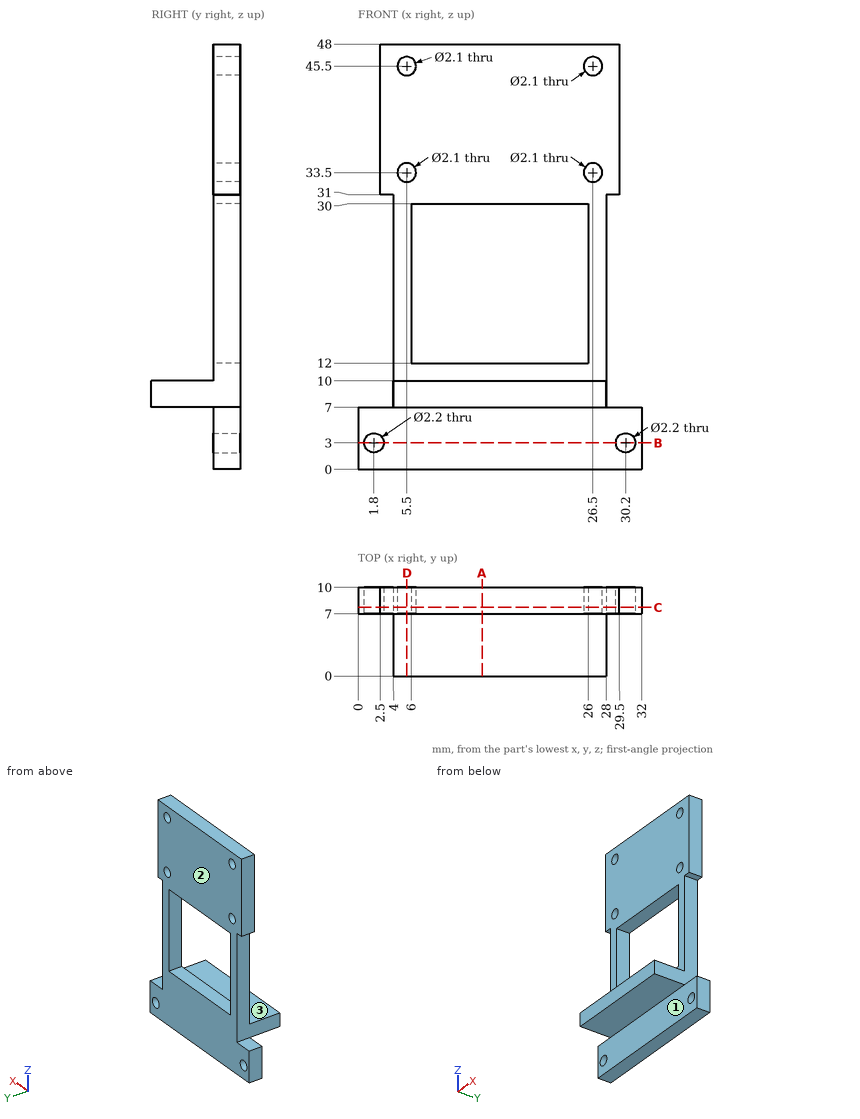
Part print with two shaded views. Sizes in mm from the minimum x, y, z corner. A direction names the side the tool comes from. Round coordinates to 2 decimals unless told otherwise and drop trailing zeros. Write each loop counter-clockwise with the first axis right and the second up, starting at its lowest first coordinate (ties: lowest second). Pieces come first, ordered by that corner, then holes. Notation, with made-up numbers: M 36.5,82.5 L 85.5,82.5 A5 cw 85.5,86.5 Z; hole C -4.5,68.5 d1. An arc over 180 degrees is marked long. Put each result on its own line as item: value. Start each with the question number.
1) Saw through at C-C, the plane y = 7.75. Write the cut outline in (x, z).
2) Pin check, flat tips, straight feed: pin 1 Ø1.7 at (x, z) = (26.5, 45.5) entering from -Y; pin 2 Ø5 at (y, z) = (8.5, 41.5) entering from +X; pin 3 Ø3.5 at (x, y) = (11.5, 2) entering from +Z; pin 4 Ø13.5 at (x, z) = (19, 24.5) entering from -Y. Stop position of each tip, or through.
3) Drill centre lines: probe 1 along Z at (x, y) = (26.5, 8); probe 2 along X at (y, z) = (8.3, 3); probe 3 along X at (y, z) = (8.3, 33.5). Where is each one in solid material? Low to high. Write a range as [from, to].
4) 3-axis set-ups, long thin cutter, end or side, ignore diameter. For the marked faces 1, 2 and 3: which of +Z, -Z, +X, -X, +Y, -Y reach the whole face in a straight line?
5) Saw through at A-A, the plane x = 14. Write the cut outline in (y, z).
6) Saw through at D-D, the plane x = 5.5. Write the cut outline in (y, z), and give its area (3 significant figures).
7) Saw through at B-B, the plane z = 3. Write the cut outline in (x, y).
Resolved:
1. outline: M 0,0 L 32,0 L 32,7 L 28,7 L 28,31 L 29.5,31 L 29.5,48 L 2.5,48 L 2.5,31 L 4,31 L 4,7 L 0,7 Z; hole C 1.8,3 d2.2; hole C 5.5,33.5 d2.1; hole C 5.5,45.5 d2.1; hole M 6,12 L 26,12 L 26,30 L 6,30 Z; hole C 26.5,33.5 d2.1; hole C 26.5,45.5 d2.1; hole C 30.2,3 d2.2
2. pin 1: through
2. pin 2: x = 29.5
2. pin 3: z = 10
2. pin 4: y = 7
3. probe 1: [0, 32.45], [34.55, 44.45], [46.55, 48]
3. probe 2: [0, 0.7], [2.9, 29.1], [31.3, 32]
3. probe 3: [2.5, 4.45], [6.55, 25.45], [27.55, 29.5]
4. face 1: -Z, +X, -X, -Y
4. face 2: +Z, -Z, +X, -X, +Y
4. face 3: +Z, +X, -X, -Y
5. outline: M 0,7 L 7,7 L 7,0 L 10,0 L 10,12 L 7,12 L 7,10 L 0,10 Z; M 7,30 L 10,30 L 10,48 L 7,48 Z
6. outline: M 0,7 L 7,7 L 7,0 L 10,0 L 10,32.45 L 7,32.45 L 7,10 L 0,10 Z; M 7,34.55 L 10,34.55 L 10,44.45 L 7,44.45 Z; M 7,46.55 L 10,46.55 L 10,48 L 7,48 Z
6. area: 152 mm²
7. outline: M 0,7 L 0.7,7 L 0.7,10 L 0,10 Z; M 2.9,7 L 29.1,7 L 29.1,10 L 2.9,10 Z; M 31.3,7 L 32,7 L 32,10 L 31.3,10 Z
